Autodesk Inventor part; units mm, degrees
ref_plane "YZ Plane" through (0, 0, 0) normal (1, 0, 0) x (0, 1, 0)
ref_plane "XZ Plane" through (0, 0, 0) normal (0, 1, 0) x (-1, 0, 0)
ref_plane "XY Plane" through (0, 0, 0) normal (0, 0, 1) x (1, 0, 0)
sketch "Эскиз1" plane through (0, 0, 0) normal (0, 1, 0) x (-1, 0, 0)
  line L0 (12.5, 12.5) -> (-12.5, 12.5)
  line L1 (-12.5, 12.5) -> (-12.5, -12.5)
  line L2 (-12.5, -12.5) -> (12.5, -12.5)
  line L3 (12.5, -12.5) -> (12.5, 12.5)
  line L4 (12.5, 12.5) -> (-12.5, -12.5) construction
  point P0 (0, 0)
  point P1 (0, 0)
  dimension "d0" = 25
  dimension "d1" = 25
extrude "Выдавливание1" add sketch "Эскиз1" along normal blind 6.3
sketch "Эскиз2" plane through (0, 6.3, 0) normal (0, 1, 0) x (1, 0, 0)
  line L0 (-10.65, -10.65) -> (10.65, -10.65)
  line L1 (10.65, -10.65) -> (10.65, 10.65)
  line L2 (10.65, 10.65) -> (-10.65, 10.65)
  line L3 (-10.65, 10.65) -> (-10.65, -10.65)
  line L4 (-10.65, -10.65) -> (10.65, 10.65) construction
  line L5 (10.65, -10.65) -> (-10.65, 10.65) construction
  line L6 (-12.5, 12.5) -> (-12.5, -12.5)
  point P0 (0, 0)
  dimension "d4" = 1.85
extrude "Выдавливание2" cut sketch "Эскиз2" against normal blind 1.2
sketch "Эскиз3" plane through (0, 5.1, 0) normal (0, 1, 0) x (1, 0, 0)
  line L0 (5, -9.75) -> (-5, -9.75)
  line L1 (-5, -9.75) -> (-5, 10.05)
  line L2 (-5, 10.05) -> (5, 10.05)
  line L3 (5, 10.05) -> (5, -9.75)
  line L4 (10.65, -10.65) -> (-10.65, -10.65)
  line L5 (0, -10.65) -> (0, 6.083) construction
  point P0 (0, 0)
  point P1 (0, -9.75)
  dimension "d7" = 10
  dimension "d8" = 19.8
  dimension "d9" = 0.9
extrude "Выдавливание3" cut sketch "Эскиз3" against normal blind 1.4
fillet "Сопряжение1" radius 1 2 edges at (-5, 5.1, -0.15) (5, 5.1, -0.15)
sketch "Эскиз6" plane through (0, 5.1, 0) normal (0, 1, 0) x (1, 0, 0)
  circle A0 centre (-9.3, 2) radius 0.4
  line L0 (-10.65, -10.65) -> (-10.65, 10.65)
  line L1 (-10.65, 10.65) -> (10.65, 10.65)
  circle A1 centre (-9.3, -8.7) radius 0.4
  line L2 (10.65, -10.65) -> (-10.65, -10.65)
  line L3 (0, -15.7072) -> (0, 17.6357) construction
  circle A2 centre (9.3, 2) radius 0.4
  circle A3 centre (9.3, -8.7) radius 0.4
  point P0 (0, 0)
  dimension "d21" = 0.8
  dimension "d22" = 1.35
  dimension "d23" = 8.65
  dimension "d24" = 0.8
  dimension "d25" = 1.35
  dimension "d26" = 1.55
extrude "Выдавливание6" add sketch "Эскиз6" along normal blind 1.2
sketch "Эскиз7" plane through (0, 3.7, 0) normal (0, 1, 0) x (1, 0, 0)
  circle A0 centre (0, -3.8434) radius 4
  point P0 (0, 0)
  dimension "d29" = 8
properties part number "Camera"
Design review of the part built by this model. Coordinates are the model's own, in mm. A direction names the side the tool comes from. Round coordinates to 2 decimals unless told otherwise and drop trailing zeros. Order: outer loops, then holes, each group sorted by start corner. A loop starts at its lowest first (then second) coordinate and runs counter-clockwise, first axis right, second up. Notation, with made-up numbers: (28, 12.25) - (63, 12.25) arc R29 cw to (63, 36.25) - close; hole circle Ø3 at (14, 15.25). An arc over 180 degrees is marked (long way). Return JSON: item names as keys, results as strings.
Q1. Machinability: for faces 4 (the flat face through (0, 4, 9.75)), 5 (the flat face through (9.3, 6.3, 8.7)), which of the approach directions +Z, -Z, +X, -X, +Y, -Y give a long, thin tool a straight path to every point of the face, cutting with its end or side? Answer none if there is none.
Computed values:
{"face 4": "+Y", "face 5": "+Z, -Z, +X, -X, +Y"}
Q2. For pin 1 Ø3 at (x, z) = (-1, -2.5) entering from +Y, flat-tipped, find the tip position at first contact; note if it passes through.
Computed values:
{"pin 1": "stops at y = 3.7"}
Q3. Consider section D-D on x = 1.75. Write out the cut boundary in (y, z).
Computed values:
{"outline": "(0, -12.5) - (6.3, -12.5) - (6.3, -10.65) - (5.1, -10.65) - (5.1, -10.05) - (3.7, -10.05) - (3.7, 9.75) - (5.1, 9.75) - (5.1, 10.65) - (6.3, 10.65) - (6.3, 12.5) - (0, 12.5) - close"}
Q4. Consider section A-A on y = 5.75. Write out the cut boundary in (x, z).
Computed values:
{"outline": "(-12.5, -12.5) - (12.5, -12.5) - (12.5, 12.5) - (-12.5, 12.5) - close; circle Ø0.8 at (-9.3, -2); circle Ø0.8 at (-9.3, 8.7); circle Ø0.8 at (9.3, -2); circle Ø0.8 at (9.3, 8.7); hole (-10.65, -10.65) - (10.65, -10.65) - (10.65, 10.65) - (-10.65, 10.65) - close"}
Q5. Consider section C-C on z = -3. Write out the cut boundary in (x, y).
Computed values:
{"outline": "(-12.5, 0) - (12.5, 0) - (12.5, 6.3) - (10.65, 6.3) - (10.65, 5.1) - (6, 5.1) arc R1 ccw to (5, 4.1) - (5, 3.7) - (-5, 3.7) - (-5, 4.1) arc R1 ccw to (-6, 5.1) - (-10.65, 5.1) - (-10.65, 6.3) - (-12.5, 6.3) - close"}
Q6. The part is to be moulded in two halves that separate along X. For faces 1 (the flat face through (0, 4, -10.05)), 2 (the flat face through (-9.3, 6.3, 8.7)), 3 (the flat face through (-12.5, 3, 0)), say which applies: pulls with the +X half, pulls with the -X half, needs draft (parallel to the pull), parting line crosses it, or undercut.
Computed values:
{"face 1": "undercut", "face 2": "needs draft", "face 3": "pulls with the -X half"}
Q7. Consider section B-B on x = -9.3. Write out the cut boundary in (y, z).
Computed values:
{"outline": "(0, -12.5) - (6.3, -12.5) - (6.3, -10.65) - (5.1, -10.65) - (5.1, -2.4) - (6.3, -2.4) - (6.3, -1.6) - (5.1, -1.6) - (5.1, 8.3) - (6.3, 8.3) - (6.3, 9.1) - (5.1, 9.1) - (5.1, 10.65) - (6.3, 10.65) - (6.3, 12.5) - (0, 12.5) - close"}
Q8. Wall thickness on L1, parallel to Z at x = 0.25, y = 5; L2, parallel to Y at x = 10, z = 1.5; L3, parallel to X at y = 3.75, z = -9.25: over which ranges is each line inside the solid? List them lowest first. Write a range as [from, to].
Computed values:
{"L1": "z = [-12.5, -10.05], [9.75, 12.5]", "L2": "y = [0, 5.1]", "L3": "x = [-12.5, -5], [5, 12.5]"}
